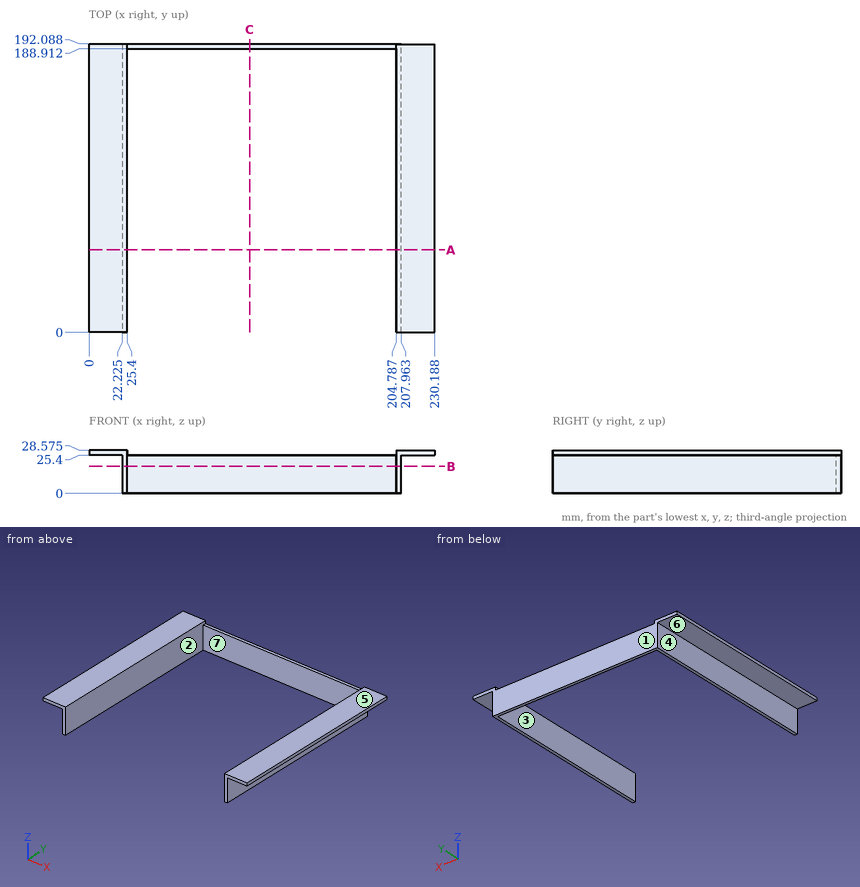
The drawing under review shows one solid part. Ordinate dimensions are in mm from its lowest x, y, z. A direction names the side the tool comes from. Round coordinates to 2 decimals unless told otherwise and drop trailing zeros. Loops run counter-clockwise (first coordinate to the right, second up) from the corner with the lowest first, then second, coordinate; pieces in that order, holes last. Notation, with made-up numbers: (-28.75, 22.5) -> (29.25, 22.5) arc R24 cw to (29.25, 44.5) -> close; hole circle Ø6 at (-35.75, 58.25). An arc over 180 degrees is marked (long way). Answer in a Markdown table with one row per item.
1) For pin 1 Ø11 at (x, y) = (223, 130) entering from -Z; pin 2 Ø2.5 at (x, y) = (113.5, 190.5) entering from +Z; pin 3 Ø5 at (x, z) = (72, 20) entering from -Y, all flat-tipped, find the tip position at first contact; note any pin that passes through.
Taken from the geometry:
| item | result |
|---|---|
| pin 1 | stops at z = 25.4 |
| pin 2 | stops at z = 25.4 |
| pin 3 | stops at y = 188.91 |
2) Tool access review of the marked faces 5, 6 and 7: name each direction out of +Z, -Z, +X, -X, +Y, -Y from which nothing blocks a thin tool from reaching the whole face with its end or side.
Taken from the geometry:
| item | result |
|---|---|
| face 5 | +Z, +X, -X, +Y, -Y |
| face 6 | -Z, -X, +Y, -Y |
| face 7 | +Z, -Z, -Y |
3) Wall thickness on line 1 along X through (y, z) = (8.5, 17.25) (1 decimal); line 2 along Y through (x, z) = (82.5, 6.75); line 3 along X through (y, z) = (22, 26): over which ranges is each line inside the solid? List them lowest first.
Taken from the geometry:
| item | result |
|---|---|
| line 1 | x = 22.2 to 25.4, 204.8 to 208 |
| line 2 | y = 188.91 to 192.09 |
| line 3 | x = 0 to 25.4, 204.79 to 230.19 |
4) Consider section B-B, the plane z = 18. Write out the cut boundary in (x, y) (1 decimal).
Taken from the geometry:
| item | result |
|---|---|
| outline | (22.2, 0) -> (25.4, 0) -> (25.4, 188.9) -> (204.8, 188.9) -> (204.8, 0) -> (208, 0) -> (208, 192.1) -> (22.2, 192.1) -> close |
5) Draft analysis for pull direction X (two halves, no side actions). For the marked faces 1, 2, 3 and 4, state which applies: pulls with the +X half, pulls with the -X half, needs draft (parallel to the pull), parting line crosses it, or undercut.
Taken from the geometry:
| item | result |
|---|---|
| face 1 | needs draft |
| face 2 | undercut |
| face 3 | undercut |
| face 4 | pulls with the -X half |
6) Consider section A-A, the plane y = 55. Write out the cut boundary in (x, z) (1 decimal).
Taken from the geometry:
| item | result |
|---|---|
| outline | (0, 25.4) -> (22.2, 25.4) -> (22.2, 0) -> (25.4, 0) -> (25.4, 28.6) -> (0, 28.6) -> close; (204.8, 0) -> (208, 0) -> (208, 25.4) -> (230.2, 25.4) -> (230.2, 28.6) -> (204.8, 28.6) -> close |
7) Consider section C-C, the plane x = 107. Write out the cut boundary in (y, z).
Taken from the geometry:
| item | result |
|---|---|
| outline | (188.91, 0) -> (192.09, 0) -> (192.09, 25.4) -> (188.91, 25.4) -> close |
